The model under review builds one solid part; all positions refer to its coordinate system, in mm. Face numbers are marked on the shaded views. Round coordinates to 2 decimals unless told otherwise and drop trailing zeros. Loops run counter-clockwise (first coordinate to the right, second up) from the corner with the lowest first, then second, coordinate; pieces in that order, holes last. Notation, with made-up numbers: (-14.75, 12.25) -> (7.25, 12.25) arc R5 ccw to (7.25, 18.25) -> close; hole circle Ø1 at (-32, -13). An arc over 180 degrees is marked (long way). Use a Markdown table: item, result. Add a question column.
1) Wall thickness on probe 1 along Z at (x, y) = (0, 8) (3 decimals); probe 2 along X at (y, z) = (8.2, 25) (3 decimals); probe 3 along X at (y, z) = (6.7, 25) (3 decimals): over which ranges is each line inside the solid? List them lowest first.
2) Insertion check: pin 1 (2 mm diameter, centred on x = 2, z = 39, fed in from -Y); pin 2 (5.5 mm diameter, centred on x = 0, z = 25, fed in from +Y). Each pin has a flat end and moves straight along its axis. Give the tip position at first contact, or say it passes through.
3) Consider section A-A on x = 0. Give the boundary of the cut face in (y, z) (3 decimals).
4) Mouldability with a two-part tool opening along X and no side actions: class the marked faces 1, 2 and 3 as released by +X, released by -X, zero draft, split by the parting line, or undercut.
5) Consider section B-B on z = 31. Give the boundary of the cut face in (x, y), plus the area to 3 significant figures.
6) Consider section D-D on y = 7.25. Give the boundary of the cut face in (x, z) (3 decimals).
7) Consider section C-C on z = 25. Give the boundary of the cut face in (x, y) (3 decimals), plus the area to 3 significant figures.
from build123d import *

# Parameters (mm, degrees)
BOSS_EXTRUDE1_DEPTH = 50
SKETCH3_R           = 2.425
CUT_EXTRUDE1_DEPTH  = 51.547558199


with BuildPart() as part:
    # Sketch2 → Boss-Extrude1 (new body)
    with BuildSketch(Plane.XY):
        with BuildLine():
            Line((-5.290927929, 9.35), (5.290927929, 9.35))
            ThreePointArc((5.290927929, 9.35), (5.748105268, 9.052457111), (5.661163141, 8.513955526))
            Line((5.661163141, 8.513955526), (3.289191157, 5.900648009))
            ThreePointArc((3.289191157, 5.900648009), (3.202240303, 5.824685234), (3.100183828, 5.770691994))
            Line((3.100183828, 5.770691994), (0.724911529, 4.846947106))
            ThreePointArc((0.724911529, 4.846947106), (0, 4.710949058), (-0.724911529, 4.846947106))
            Line((-0.724911529, 4.846947106), (-3.100183828, 5.770691994))
            ThreePointArc((-3.100183828, 5.770691994), (-3.202240303, 5.824685234), (-3.289191157, 5.900648009))
            Line((-3.289191157, 5.900648009), (-5.661163141, 8.513955526))
            ThreePointArc((-5.661163141, 8.513955526), (-5.748105268, 9.052457111), (-5.290927929, 9.35))
        make_face()
    extrude(amount=BOSS_EXTRUDE1_DEPTH)

    # Sketch3 → Cut-Extrude1 (cut, through all)
    with BuildSketch(Plane(origin=(0, 9.35, 0), x_dir=(1, 0, 0), z_dir=(0, 1, 0))):
        with Locations(Location((0, -25, 0), (0, 0, 270))):
            Circle(SKETCH3_R)
    extrude(amount=-CUT_EXTRUDE1_DEPTH, mode=Mode.SUBTRACT)


solid = part.part
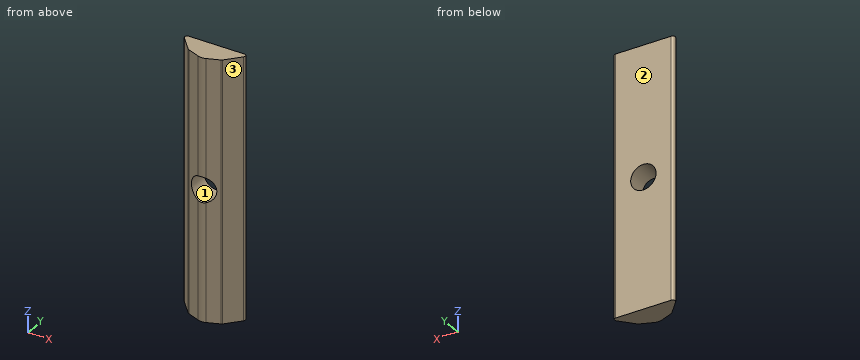
Result set:
| question | item | result |
|---|---|---|
| 1 | probe 1 | 0 to 22.575, 27.425 to 50 |
| 1 | probe 2 | -5.376 to -2.425, 2.425 to 5.376 |
| 1 | probe 3 | -4.015 to -2.425, 2.425 to 4.015 |
| 2 | pin 1 | y = 4.95 |
| 2 | pin 2 | y = 9.35 |
| 3 | outline | (4.711, 0) -> (9.35, 0) -> (9.35, 22.575) -> (4.711, 22.575) -> close; (4.711, 27.425) -> (9.35, 27.425) -> (9.35, 50) -> (4.711, 50) -> close |
| 4 | face 1 | undercut |
| 4 | face 2 | zero draft |
| 4 | face 3 | released by +X |
| 5 | outline | (-5.66, 8.51) -> (-3.29, 5.9) arc R0.5 ccw to (-3.1, 5.77) -> (-0.72, 4.85) arc R2 ccw to (0.72, 4.85) -> (3.1, 5.77) arc R0.5 ccw to (3.29, 5.9) -> (5.66, 8.51) arc R0.5 ccw to (5.29, 9.35) -> (-5.29, 9.35) arc R0.5 ccw to start |
| 5 | area | 37.4 mm2 |
| 6 | outline | (-4.514, 0) -> (4.514, 0) -> (4.514, 50) -> (-4.514, 50) -> close; hole circle Ø4.85 at (0, 25) |
| 7 | outline | (-5.661, 8.514) -> (-3.289, 5.901) arc R0.5 ccw to (-3.1, 5.771) -> (-2.425, 5.508) -> (-2.425, 9.35) -> (-5.291, 9.35) arc R0.5 ccw to start; (2.425, 5.508) -> (3.1, 5.771) arc R0.5 ccw to (3.289, 5.901) -> (5.661, 8.514) arc R0.5 ccw to (5.291, 9.35) -> (2.425, 9.35) -> close |
| 7 | area | 16.6 mm2 |
